```python
from build123d import *

# Parameters (mm, degrees)
CHAMFER1_SIZE = 0.5
FILLET2_R     = 1


with BuildPart() as part:
    # Sketch1 → Revolve1 (revolve)
    with BuildSketch(Plane.XY, mode=Mode.PRIVATE) as revolve1_sk:
        with BuildLine():
            Line((5, -2.5), (6.350510257, -2.5))
            ThreePointArc((6.350510257, -2.5), (8.8, -3.5), (11.249489743, -2.5))
            Line((11.249489743, -2.5), (13, -2.5))
            Line((13, -2.5), (13, -5.5))
            Line((13, -5.5), (5, -5.5))
            Line((5, -5.5), (5, -2.5))
        make_face()
    revolve(revolve1_sk.sketch.rotate(Axis((0, 5.5, 0), (0, -1, 0)), 180), axis=Axis((0, 5.5, 0), (0, -1, 0)))

    # Chamfer1
    chamfer1_edges = [part.edges().sort_by_distance(p)[0] for p in [
        (5, -2.5, 0),
        (13, -2.5, 0),
    ]]
    chamfer(chamfer1_edges, length=CHAMFER1_SIZE)

    # Fillet2
    fillet2_edges = [part.edges().sort_by_distance(p)[0] for p in [
        (13, -5.5, 0),
        (5, -5.5, 0),
    ]]
    fillet(fillet2_edges, radius=FILLET2_R)


solid = part.part
```
The listing builds one solid part. Answer for the finished solid, in the listing's coordinates (mm). Round coordinates to 2 decimals unless told otherwise and drop trailing zeros. Loops run counter-clockwise (first coordinate to the right, second up) from the corner with the lowest first, then second, coordinate; pieces in that order, holes last. Notation, with made-up numbers: (36, -34) -> (82, -34) arc R14 cw to (82, -22) -> close; hole circle Ø11 at (-32, -33.75). An arc over 180 degrees is marked (long way). Use one line per item in the form item = value.
1. For a pull along Z with two mould halves and no side action, classify faces 1 (the cylindrical face through (10.316, -3.76, 7.91)), 2 (the cylindrical face through (5, -4, 0)), 3 (the flat face through (-5, -2.5, -3)) as released by +Z, released by -Z, zero draft, split by the parting line, or undercut.
Answer key:
face_1 = split by the parting line
face_2 = undercut
face_3 = zero draft
2. The part is cut by section C-C on y = -3.9. Determine the outline of the cut face in (x, z).
Answer key:
outline = circle Ø26 at (0, 0); hole circle Ø10 at (0, 0)
3. The part is cut by section B-B on x = 0. Determine the outline of the cut face in (y, z).
Answer key:
outline = (-5.5, -12) arc R1 ccw to (-4.5, -13) -> (-3, -13) -> (-2.5, -12.5) -> (-2.5, -11.25) arc R3.5 cw to (-2.5, -6.35) -> (-2.5, -5.5) -> (-3, -5) -> (-4.5, -5) arc R1 ccw to (-5.5, -6) -> close; (-5.5, 6) arc R1 ccw to (-4.5, 5) -> (-3, 5) -> (-2.5, 5.5) -> (-2.5, 6.35) arc R3.5 cw to (-2.5, 11.25) -> (-2.5, 12.5) -> (-3, 13) -> (-4.5, 13) arc R1 ccw to (-5.5, 12) -> close
4. Find the intervals of material crossed by probe 1 along Z at (x, y) = (0, -4); probe 2 along X at (y, z) = (-3, -0.5); probe 3 along Z at (x, y) = (3, -3.15), in increasing order. Write a range as [from, to].
Answer key:
probe_1 = [-13, -5], [5, 13]
probe_2 = [-12.99, -10.59], [-6.98, -4.97], [4.97, 6.98], [10.59, 12.99]
probe_3 = [-12.65, -9.88], [-6.63, -4], [4, 6.63], [9.88, 12.65]
5. Flat-ended cylindrical pins translate along their axes: pin 1 Ø1.5 at (x, z) = (-0.5, -5.5) entering from -Y; pin 2 Ø1 at (x, y) = (2, -4) entering from +Z. Find the tip coordinate at first contact, or state that the pin passes through.
Answer key:
pin_1 = -5.5
pin_2 = 12.91
6. The part is cut by section A-A on z = 0. Determine the outline of the cut face in (x, y), and give its area (3 significant figures).
Answer key:
outline = (-13, -4.5) arc R1 ccw to (-12, -5.5) -> (-6, -5.5) arc R1 ccw to (-5, -4.5) -> (-5, -3) -> (-5.5, -2.5) -> (-6.35, -2.5) arc R3.5 cw to (-11.25, -2.5) -> (-12.5, -2.5) -> (-13, -3) -> close; (5, -4.5) arc R1 ccw to (6, -5.5) -> (12, -5.5) arc R1 ccw to (13, -4.5) -> (13, -3) -> (12.5, -2.5) -> (11.25, -2.5) arc R3.5 cw to (6.35, -2.5) -> (5.5, -2.5) -> (5, -3) -> close
area = 39.9 mm²
